Work out the finished part from the listing and answer in its coordinate system (mm). Coordinates: 2 decimals unless noted, no trailing zeros. Order: outer loops, then holes, each group sorted by start corner. A loop starts at its lowest first (then second) coordinate and runs counter-clockwise, first axis right, second up.
1. A flat-ended cylindrical pin translates along its axis: pin 1 Ø8 at (y, z) = (-25.4, -19.05) entering from -X. Find the tip coordinate at first contact, or state that the pin passes through.
2. The part is cut by section B-B, the plane z = 57.15. Give the vertices of the cut face in (x, y).
3. The part is cut by section C-C, the plane z = -19.05. Give the vertices of the cut face in (x, y), then the cut area to 3 significant figures.
4. The part is cut by section A-A, the plane y = 25.4. Give the vertices of the cut face in (x, z).
5. Determine the mould class of faces 1 (the cylindrical face through (3.219, 27.082, -17.215)), 2 (the flat face through (3, 0, 63.5)), 3 (the flat face through (0, 0, 1)) for opening direction Z: +Z half, -Z half, draft (parallel to the pull), parting line (faces both ways), or undercut.
6. Find the intervals of material crossed by probe 1 along Y at (x, z) = (2.25, -57.15); probe 2 along Z at (x, y) = (5.25, -21); probe 3 along Y at (x, z) = (1.25, 5), in increasing order.
```python
from build123d import *

# Parameters (mm, degrees)
SKETCH1_W                      = 127
SKETCH1_H                      = 63.5
BOSS_EXTRUDE1_DEPTH            = 6.35
F_9_0_196_DIAMETER_HOLE1_D     = 4.9784
F_9_0_196_DIAMETER_HOLE1_DEPTH = 70.104
F_9_0_196_DIAMETER_HOLE1_TIP   = 1.495662253
F_9_0_196_DIAMETER_HOLE2_D     = 4.9784
F_9_0_196_DIAMETER_HOLE2_DEPTH = 70.104
F_9_0_196_DIAMETER_HOLE2_TIP   = 1.495662253


with BuildPart() as part:
    # Sketch1 → Boss-Extrude1 (new body)
    with BuildSketch(Plane(origin=(0, 0, 0), x_dir=(0, 0, -1), z_dir=(1, 0, 0))):
        Rectangle(SKETCH1_W, SKETCH1_H)
    extrude(amount=BOSS_EXTRUDE1_DEPTH)

    # #9 (0.196) Diameter Hole1
    with Locations(Plane.ZY):
        with Locations((57.15, -22.225), (6.35, -22.225)):
            Hole(F_9_0_196_DIAMETER_HOLE1_D / 2, depth=F_9_0_196_DIAMETER_HOLE1_DEPTH)
            with Locations((0, 0, -(F_9_0_196_DIAMETER_HOLE1_DEPTH + F_9_0_196_DIAMETER_HOLE1_TIP / 2))):  # 118° drill point
                Cone(0, F_9_0_196_DIAMETER_HOLE1_D / 2, F_9_0_196_DIAMETER_HOLE1_TIP, mode=Mode.SUBTRACT)

    # #9 (0.196) Diameter Hole2
    with Locations(Plane.ZY):
        with Locations((-57.15, -25.4), (-19.05, -25.4), (-19.05, 25.4), (-57.15, 25.4)):
            Hole(F_9_0_196_DIAMETER_HOLE2_D / 2, depth=F_9_0_196_DIAMETER_HOLE2_DEPTH)
            with Locations((0, 0, -(F_9_0_196_DIAMETER_HOLE2_DEPTH + F_9_0_196_DIAMETER_HOLE2_TIP / 2))):  # 118° drill point
                Cone(0, F_9_0_196_DIAMETER_HOLE2_D / 2, F_9_0_196_DIAMETER_HOLE2_TIP, mode=Mode.SUBTRACT)


solid = part.part
```
Geometry says:
1. pin 1: stops at x = 0
2. outline: (0, -31.75) - (6.35, -31.75) - (6.35, -24.71) - (0, -24.71) - close; (0, -19.74) - (6.35, -19.74) - (6.35, 31.75) - (0, 31.75) - close
3. outline: (0, -31.75) - (6.35, -31.75) - (6.35, -27.89) - (0, -27.89) - close; (0, -22.91) - (6.35, -22.91) - (6.35, 22.91) - (0, 22.91) - close; (0, 27.89) - (6.35, 27.89) - (6.35, 31.75) - (0, 31.75) - close
3. area: 340 mm2
4. outline: (0, -63.5) - (6.35, -63.5) - (6.35, -59.64) - (0, -59.64) - close; (0, -54.66) - (6.35, -54.66) - (6.35, -21.54) - (0, -21.54) - close; (0, -16.56) - (6.35, -16.56) - (6.35, 63.5) - (0, 63.5) - close
5. face 1: undercut
5. face 2: +Z half
5. face 3: draft
6. probe 1: y = -31.75 to -27.89, -22.91 to 22.91, 27.89 to 31.75
6. probe 2: z = -63.5 to 4.18, 8.52 to 54.98, 59.32 to 63.5
6. probe 3: y = -31.75 to -24.32, -20.13 to 31.75
